Drawing for the job (mm, zero at the part's lowest x, y, z). A direction names the side the tool comes from. Give positions to 0.01 mm unless a question says otherwise; leave off trailing zeros. Write each loop counter-clockwise with the first axis right and the second up, starting at its lowest first coordinate (ties: lowest second). Pieces come first, ordered by that corner, then holes. Notation, with made-up numbers: (26, -12) - (36, -12) arc R14 ccw to (36, -2) - close; hole circle Ø4 at (37.5, 26). An arc over 180 degrees is marked (long way). Write item = value, one per line. Start each with the question number.
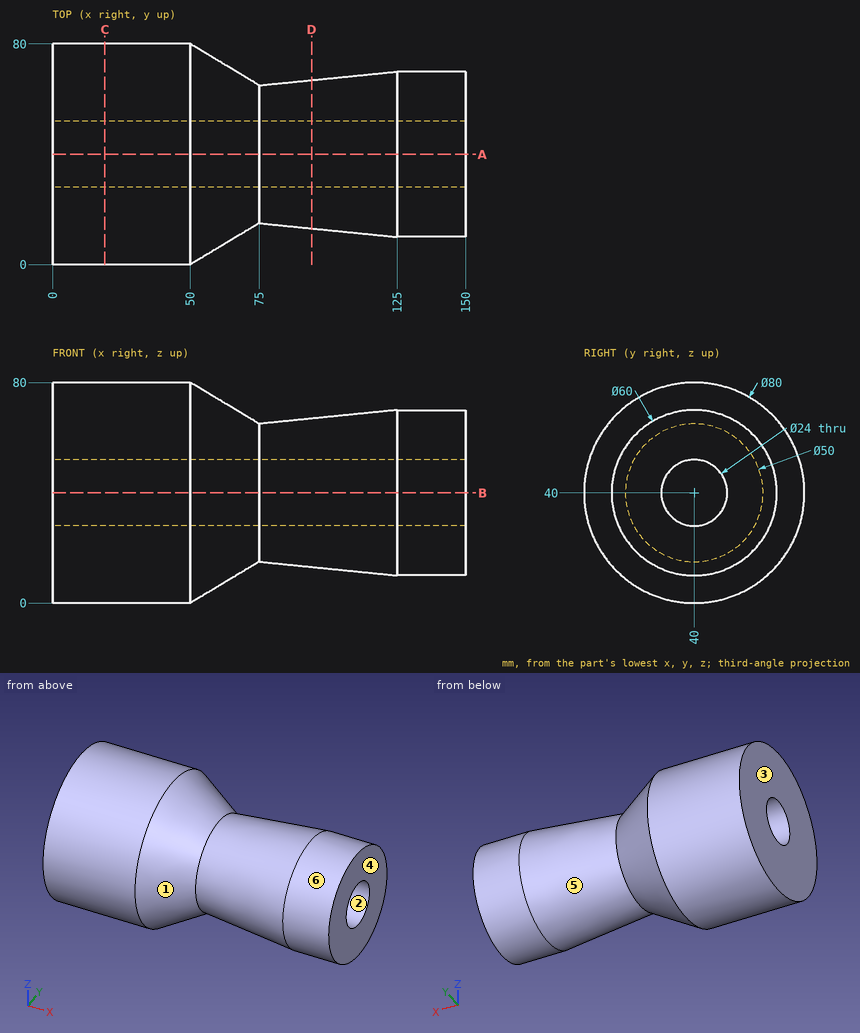
1. Cut at C-C (x = 19). Give the cut face in (y, z).
2. Pin check, flat tips, straight feed: pin 1 Ø12 at (x, z) = (23.5, 33) entering from -Y; pin 2 Ø5 at (x, z) = (37.5, 51.5) entering from -Y; pin 3 Ø1.5 at (x, z) = (65, 32) entering from -Y. Stop position of each tip, or through.
3. Cut at A-A (y = 40). Give the cut face in (x, z), then the cut area to 4 significant figures.
4. Tool access for the marked faces 1 and 2: list every direction of +Z, -Z, +X, -X, +Y, -Y with a clear straight run to the whole face (end or side of a thin tool).
5. Wall check: line 1 along Z through (x, y) = (44, 40); line 2 along Y through (x, z) = (94.5, 29); line 3 along Y through (x, z) = (115, 40). Give the ranges that are in metal, low to high.
6. Cut at D-D (x = 94). Give the cut face in (y, z), then the cut area to 3 significant figures.
7. Mould opens along X. For the marked faces 3, 4, 5 and 6 say: +X half, -X half, draft (parallel to the pull), parting line (faces both ways), or undercut.
Output:
q1.outline = circle Ø80 at (40, 40); hole circle Ø24 at (40, 40)
q2.pin_1 = 0.01
q2.pin_2 = 1.03
q2.pin_3 = 9.55
q3.outline = (0, 0) - (50, 0) - (75, 15) - (125, 10) - (150, 10) - (150, 28) - (0, 28) - close; (0, 52) - (150, 52) - (150, 70) - (125, 70) - (75, 65) - (50, 80) - (0, 80) - close
q3.area = 6,275 mm2
q4.face_1 = none
q4.face_2 = +X, -X
q5.line_1 = 0 to 28, 52 to 80
q5.line_2 = 15.4 to 35.2, 44.8 to 64.6
q5.line_3 = 11 to 28, 52 to 69
q6.outline = circle Ø53.8 at (40, 40); hole circle Ø24 at (40, 40)
q6.area = 1,820 mm2
q7.face_3 = -X half
q7.face_4 = +X half
q7.face_5 = undercut
q7.face_6 = draft
